Here's how the part is built. I have some questions about the finished solid (model axes, mm). A direction names the side the tool comes from. Give positions to 0.01 mm unless a question says otherwise; leave off trailing zeros. Loops run counter-clockwise (first coordinate to the right, second up) from the corner with the lowest first, then second, coordinate; pieces in that order, holes last. Notation, with made-up numbers: (29, -24.5) - (69, -24.5) arc R27 ccw to (69, 7.5) - close; hole circle Ø11 at (-13.75, -4). An arc over 180 degrees is marked (long way). Use a Markdown table: item, result.
from build123d import *

# Parameters (mm, degrees)
F1_DEPTH = 20
F2_R     = 2
F3_DEPTH = 25
F4_R     = 4.99999


# Not quite as in the source:
# - a fillet or chamfer is up to 0.001 mm smaller than in the source, because OpenCascade refuses the exact size


with BuildPart() as f1:
    # F0 (on Top) → F1 (new body)
    with BuildSketch(Plane.XY):
        Polygon((-38, 33), (0, 33), (0, 37), (-42, 37), (-42, 4), (-57, 4), (-57, 0), (-38, 0), align=None)
        Polygon((0, 37), (0, 33), (38, 33), (38, 0), (57, 0), (57, 4), (42, 4), (42, 37), align=None)
    extrude(amount=F1_DEPTH)

    # F2 (on face) → F3 (cut)
    with BuildSketch(Plane(origin=(0, 4, 0), x_dir=(-1, 0, 0), z_dir=(0, 1, 0))):
        with Locations((49, 10)):
            Circle(F2_R)
        with Locations((-49, 10)):
            Circle(F2_R)
    extrude(amount=-F3_DEPTH, mode=Mode.SUBTRACT)

    # F4 (radius 5 in the source; OpenCascade refuses exactly that, so slightly less here)
    f4_edges = [f1.edges().sort_by_distance(p)[0] for p in [
        (-57, 2, 20),
        (-57, 2, 0),
        (57, 2, 0),
        (57, 2, 20),
        (42, 37, 10),
        (-42, 37, 10),
        (-38, 0, 10),
        (38, 0, 10),
        (42, 4, 10),
        (-42, 4, 10),
    ]]
    fillet(f4_edges, radius=F4_R)


solid = f1.part
(1) Suppose I cut it at D-D on z = 13. Write out the boundary of the cut face in (x, y).
A:
| item | result |
|---|---|
| outline | (-57, 0) - (-43, 0) arc R5 ccw to (-38, 5) - (-38, 33) - (38, 33) - (38, 5) arc R5 ccw to (43, 0) - (57, 0) - (57, 4) - (47, 4) arc R5 cw to (42, 9) - (42, 32) arc R5 ccw to (37, 37) - (-37, 37) arc R5 ccw to (-42, 32) - (-42, 9) arc R5 cw to (-47, 4) - (-57, 4) - close |
(2) Will these pins go through, and if not, where does the flat tip stop? pin 1 (4.5 mm diameter, centred on x = 49, z = 10, fed in from +Y); pin 2 (8 mm diameter, centred on x = 33, y = 31, fed in from +Z); pin 3 (2 mm diameter, centred on y = 6, z = 12.5, fed in from +X); pin 4 (10 mm diameter, centred on y = 15.5, z = 10, fed in from +X).
A:
| item | result |
|---|---|
| pin 1 | y = 4.01 |
| pin 2 | z = 20 |
| pin 3 | x = 44 |
| pin 4 | x = 42 |
(3) On a 3-axis mill with a long thin cutter (end or side, diameter ignored), from which of +Z, -Z, +X, -X, +Y, -Y can I reach the whole of each face in a straight line? I mean faces 1 (the face through (-42, 21, 10)), 2 (the face through (-38, 19, 10)), 3 (the face through (42, 20, 10)). Say none if no direction works.
A:
| item | result |
|---|---|
| face 1 | +Z, -Z, -X, +Y |
| face 2 | +Z, -Z, -Y |
| face 3 | +Z, -Z, +X, +Y |
(4) We'd pull the mould along X, two halves only. Please class faces 4 (the face through (55, 2, 19)), 5 (the face through (1, 37, 10)), 6 (the face through (39, 2, 10)): pulls with the +X half, pulls with the -X half, needs draft (parallel to the pull), parting line crosses it, or undercut.
A:
| item | result |
|---|---|
| face 4 | pulls with the +X half |
| face 5 | needs draft |
| face 6 | undercut |
(5) If I drill on line 1 (X direction, y = 31.5, z = 15.25); line 2 (Z direction, x = -49, y = 2.55); line 3 (Y direction, x = 15.5, z = 12.5), over which ranges is the centre line in solid material (lowest first)?
A:
| item | result |
|---|---|
| line 1 | -42 to -38, 38 to 42 |
| line 2 | 0 to 8, 12 to 20 |
| line 3 | 33 to 37 |
(6) Suppose I cut it at B-B on x = 49. Write out the boundary of the cut face in (y, z).
A:
| item | result |
|---|---|
| outline | (0, 0) - (4, 0) - (4, 8) - (0, 8) - close; (0, 12) - (4, 12) - (4, 20) - (0, 20) - close |
(7) Suppose I cut it at C-C on y = 12. Write out the boundary of the cut face in (x, z).
A:
| item | result |
|---|---|
| outline | (-42, 0) - (-38, 0) - (-38, 20) - (-42, 20) - close; (38, 0) - (42, 0) - (42, 20) - (38, 20) - close |
(8) Suppose I cut it at A-A on y = 2. Write out the boundary of the cut face in (x, z), plus the area to 3 significant figures.
A:
| item | result |
|---|---|
| outline | (-57, 5) arc R5 ccw to (-52, 0) - (-39, 0) - (-39, 20) - (-52, 20) arc R5 ccw to (-57, 15) - close; (39, 0) - (52, 0) arc R5 ccw to (57, 5) - (57, 15) arc R5 ccw to (52, 20) - (39, 20) - close; hole circle Ø4 at (-49, 10); hole circle Ø4 at (49, 10) |
| area | 673 mm2 |
